```python
from build123d import *

# Parameters (mm, degrees)
SKETCH_1_R          = 15
SKETCH_1_R_2        = 10
EXTRUDE_1_DEPTH     = 30
CUT_EXTRUDE_START   = -30
CUT_EXTRUDE_1_DEPTH = 30
SKETCH_3_R          = 2.5
EXTRUDE_2_DEPTH     = 8


# Read off the part's stored shape, not the designer's step: 切除-拉伸1
with BuildPart() as part:
    # 草图1 → 凸台-拉伸1 (new body)
    # profile 1 of 3: a face of its own
    with BuildSketch(Plane.XY):
        Circle(SKETCH_1_R)
        Circle(SKETCH_1_R_2, mode=Mode.SUBTRACT)
    # profile 2 of 3: a face of its own
    with BuildSketch(Plane.XY):
        with BuildLine():
            ThreePointArc((40.902315542, 38.073888417), (39.393398282, 39.393398282), (38.073888417, 40.902315542))
            Line((38.073888417, 40.902315542), (9.097684458, 11.926111583))
            ThreePointArc((9.097684458, 11.926111583), (10.606601718, 10.606601718), (11.926111583, 9.097684458))
            Line((11.926111583, 9.097684458), (40.902315542, 38.073888417))
        make_face()
    # profile 3 of 3: a face of its own
    with BuildSketch(Plane.XY):
        with Locations((50, 50)):
            Circle(SKETCH_1_R)
        with Locations((50, 50)):
            Circle(SKETCH_1_R_2, mode=Mode.SUBTRACT)
    extrude(amount=EXTRUDE_1_DEPTH)

    # 切除-拉伸1 outline → 切除-拉伸1 (cut)
    with BuildSketch(Plane.XY.offset(30).offset(CUT_EXTRUDE_START)):
        with BuildLine():
            Line((56.261708011, 36.3694823), (43.738291989, 36.3694823))
            ThreePointArc((43.738291989, 36.3694823), (50, 35), (56.261708011, 36.3694823))
        make_face()
    extrude(amount=CUT_EXTRUDE_1_DEPTH, mode=Mode.SUBTRACT)

    # 草图3 → 凸台-拉伸2 (add)
    with BuildSketch(Plane(origin=(0, 36.369482299, 0), x_dir=(-1, 0, 0), z_dir=(0, -1, 0))):
        with Locations(Location((-49.626061582, -11.687427951, 0), (0, 0, 90))):
            Circle(SKETCH_3_R)
    extrude(amount=EXTRUDE_2_DEPTH)


solid = part.part
```
Here's how the part is built. I have some questions about the finished solid (model axes, mm). A direction names the side the tool comes from. Coordinates: 2 decimals unless noted, no trailing zeros. Write each loop counter-clockwise with the first axis right and the second up, starting at its lowest first coordinate (ties: lowest second). Pieces come first, ordered by that corner, then holes. Notation, with made-up numbers: (43, 12.5) -> (92, 12.5) arc R23 ccw to (92, 51.5) -> close; hole circle Ø7 at (-16, 23). An arc over 180 degrees is marked (long way). Use a Markdown table: item, result. Add a question column.
(1) For faces 4 (the cylindrical face through (52.105, 32.425, 12.013)), 5 (the cylindrical face through (47.83, 40.24, 14.79)), 6 (the flat face through (50, 28.369, 12)), which set-ups out of +Z, -Z, +X, -X, +Y, -Y let a thin tool reach every point of the face, with its end or its side?
(2) If we section it at C-C, the plane z = 2: Write out the boundary of the cut face in (x, y), and give its area (3 significant figures).
(3) Please list where these lines run through material, in increasing order: line 1 (Y direction, x = 0, z = 21.75); line 2 (Y direction, x = 50, z = 12.75); line 3 (X direction, y = 9, z = 13.25).
(4) If we section it at A-A, the plane x = 0: Write out the boundary of the cut face in (y, z), and give its area (3 significant figures).
(5) I'm going to push flat-ended pins straight in: P1, Ø6, axis at y = 52, z = 10.5, coming from the +X side; P2, Ø4, axis at x = 49.5, z = 12, coming from the -Y side; P3, Ø4, axis at x = 16.5, z = 13.5, coming from the +Y side; P4, Ø2, axis at x = 45, z = 27, coming from the -Y side. Where does each tip first touch, or does it pass through?
(6) If we section it at B-B, the plane y = 50: Write out the boundary of the cut face in (x, z), and give its area (3 significant figures).
(7) We'd pull the mould along X, two halves only. Please class faces 1 (the cylindrical face through (42.253, 37.155, 14.79)), 2 (the flat face through (25, 25, 30)), 3 (the cylindrical face through (54.13, 64.42, 14.79)): +X half, -X half, draft (parallel to the pull), parting line (faces both ways), or undercut.
(8) If we section it at D-D, the plane z = 12.25: Write out the boundary of the cut face in (x, y).
Outcome:
| question | item | result |
|---|---|---|
| 1 | face 4 | -Y |
| 1 | face 5 | +Z, -Z |
| 1 | face 6 | +Z, -Z, +X, -Y |
| 2 | outline | (9.1, 11.93) arc R15 ccw (long way) to (11.93, 9.1) -> (40.9, 38.07) arc R15 ccw to (43.74, 36.37) -> (56.26, 36.37) arc R15 ccw (long way) to (38.07, 40.9) -> close; hole circle Ø20 at (0, 0); hole circle Ø20 at (50, 50) |
| 2 | area | 937 mm^2 |
| 3 | line 1 | y = -15 to -10, 10 to 15 |
| 3 | line 2 | y = 28.37 to 40, 60 to 65 |
| 3 | line 3 | x = -12 to -4.36, 4.36 to 12 |
| 4 | outline | (-15, 0) -> (-10, 0) -> (-10, 30) -> (-15, 30) -> close; (10, 0) -> (15, 0) -> (15, 30) -> (10, 30) -> close |
| 4 | area | 300 mm^2 |
| 5 | P1 | stops at x = 65 |
| 5 | P2 | stops at y = 28.37 |
| 5 | P3 | stops at y = 21.33 |
| 5 | P4 | stops at y = 36.37 |
| 6 | outline | (35, 0) -> (40, 0) -> (40, 30) -> (35, 30) -> close; (60, 0) -> (65, 0) -> (65, 30) -> (60, 30) -> close |
| 6 | area | 300 mm^2 |
| 7 | face 1 | undercut |
| 7 | face 2 | draft |
| 7 | face 3 | parting line |
| 8 | outline | (9.1, 11.93) arc R15 ccw (long way) to (11.93, 9.1) -> (40.9, 38.07) arc R15 ccw to (43.74, 36.37) -> (47.19, 36.37) -> (47.19, 28.37) -> (52.06, 28.37) -> (52.06, 36.37) -> (56.26, 36.37) arc R15 ccw (long way) to (38.07, 40.9) -> close; hole circle Ø20 at (0, 0); hole circle Ø20 at (50, 50) |
